Part model, mm, in its own coordinate system. A direction names the side the tool comes from. Round coordinates to 2 decimals unless told otherwise and drop trailing zeros. Loops run counter-clockwise (first coordinate to the right, second up) from the corner with the lowest first, then second, coordinate; pieces in that order, holes last.
1) Drop flat-ended pins along their axis: P1, Ø3, axis at x = 0.15, z = -17.99, coming from the -Y side; P2, Ø3, axis at x = -2.5, z = 8, coming from the +Y side; P3, Ø1.6, axis at x = 0.15, z = 20.01, coming from the -Y side. Give the stop position or say it passes through.
2) Band-saw the part on C-C, the plane z = -1. Write the cut outline in (x, y), then the cut area to 3 significant figures.
3) Band-saw the part on B-B, the plane x = -4. Write the cut outline in (y, z), then the cut area to 3 significant figures.
4) Probe line 1 (Z direction, x = -4, y = 4.6); line 2 (Y direction, x = -1, z = 8); line 3 (X direction, y = 3.9, z = -17.5). List the from-to ranges inside material, lowest first.
5) Band-saw the part on A-A, the plane y = 4.5. Write the cut outline in (x, z).
6) 3-axis set-ups, long thin cutter, end or side, ignore diameter. For faces 4 (the flat face through (0.1, 5, 18.8)), 5 (the flat face through (0, 4, 15.007)): which of +Z, -Z, +X, -X, +Y, -Y reach the whole face in a straight line?
7) Mould opens along Z. For faces 1 (the flat face through (-1, 5, -18.1)), 2 (the cylindrical face through (0.19, 2.54, -18.99)), 3 (the flat face through (0, 2, 25.007)) say: +Z half, -Z half, draft (parallel to the pull), parting line (faces both ways), or undercut.
from build123d import *

# Parameters (mm, degrees)
SKETCH1_W           = 10
SKETCH1_H           = 48
BOSS_EXTRUDE1_DEPTH = 3.5
SKETCH2_W           = 10
SKETCH2_H           = 10
BOSS_EXTRUDE2_DEPTH = 1.5
SKETCH3_R           = 1
CUT_EXTRUDE1_DEPTH  = 5


with BuildPart() as part:
    # Sketch1 → Boss-Extrude1 (new body)
    with BuildSketch(Plane(origin=(0, 0, 0), x_dir=(1, 0, 0), z_dir=(0, 1, 0))):
        with Locations((0.145631068, -1.007103337)):
            Rectangle(SKETCH1_W, SKETCH1_H)
    extrude(amount=BOSS_EXTRUDE1_DEPTH)

    # Sketch2 → Boss-Extrude2 (add)
    with BuildSketch(Plane(origin=(0, 3.5, 0), x_dir=(1, 0, 0), z_dir=(0, 1, 0))):
        with Locations((0.145631068, 17.992896663)):
            Rectangle(SKETCH2_W, SKETCH2_H)
        with Locations((0.145631068, -20.007103337)):
            Rectangle(SKETCH2_W, SKETCH2_H)
    extrude(amount=BOSS_EXTRUDE2_DEPTH)

    # Sketch3 → Cut-Extrude1 (cut)
    with BuildSketch(Plane(origin=(0, 5, 0), x_dir=(1, 0, 0), z_dir=(0, 1, 0))):
        with Locations(Location((0.145631068, 17.992896663, 0), (0, 0, 270))):
            Circle(SKETCH3_R)
        with Locations(Location((0.145631068, -20.007103337, 0), (0, 0, 270))):
            Circle(SKETCH3_R)
    extrude(amount=-CUT_EXTRUDE1_DEPTH, mode=Mode.SUBTRACT)


solid = part.part
Reported:
1. P1: stops at y = 0
1. P2: stops at y = 3.5
1. P3: passes through
2. outline: (-4.85, 0) - (5.15, 0) - (5.15, 3.5) - (-4.85, 3.5) - close
2. area: 35.0 mm2
3. outline: (0, -22.99) - (5, -22.99) - (5, -12.99) - (3.5, -12.99) - (3.5, 15.01) - (5, 15.01) - (5, 25.01) - (0, 25.01) - close
3. area: 198 mm2
4. line 1: z = -22.99 to -12.99, 15.01 to 25.01
4. line 2: y = 0 to 3.5
4. line 3: x = -4.85 to -0.72, 1.02 to 5.15
5. outline: (-4.85, -22.99) - (5.15, -22.99) - (5.15, -12.99) - (-4.85, -12.99) - close; (-4.85, 15.01) - (5.15, 15.01) - (5.15, 25.01) - (-4.85, 25.01) - close; hole circle Ø2 at (0.15, -17.99); hole circle Ø2 at (0.15, 20.01)
6. face 4: +Z, -Z, +X, -X, +Y
6. face 5: +X, -X, +Y
7. face 1: draft
7. face 2: undercut
7. face 3: +Z half
